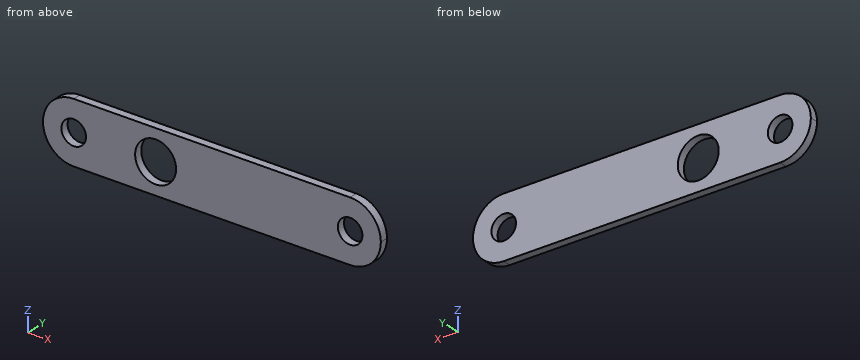
```python
from build123d import *

# Parameters (mm, degrees)
F0_W     = 82.5
F0_H     = 15
F0_R     = 3
F1_DEPTH = 1
F2_R     = 7.49999
F3_R     = 5
F4_DEPTH = 12.5


# Not quite as in the source:
# - a fillet or chamfer is up to 0.001 mm smaller than in the source, because OpenCascade refuses the exact size


with BuildPart() as f1:
    # F0 (on Front) → F1 (new body, symmetric)
    with BuildSketch(Plane.XZ):
        with Locations((33.75, 0)):
            Rectangle(F0_W, F0_H)
        Circle(F0_R, mode=Mode.SUBTRACT)
        with Locations((67.5, 0)):
            Circle(F0_R, mode=Mode.SUBTRACT)
    extrude(amount=F1_DEPTH, both=True)

    # F2 (radius 7.5 in the source; OpenCascade refuses exactly that, so slightly less here)
    f2_edges = [f1.edges().sort_by_distance(p)[0] for p in [
        (75, 0, 7.5),
        (75, 0, -7.5),
        (-7.5, 0, 7.5),
        (-7.5, 0, -7.5),
    ]]
    fillet(f2_edges, radius=F2_R)

    # F3 (on Front) → F4 (cut, symmetric)
    with BuildSketch(Plane.XZ):
        with Locations((20, 0)):
            Circle(F3_R)
    extrude(amount=F4_DEPTH, both=True, mode=Mode.SUBTRACT)


solid = f1.part
```
Check sheet for the modelled part. Datum: model origin and axes. Units: mm. Round coordinates to 2 decimals unless told otherwise and drop trailing zeros. Order: outer loops, then holes, each group sorted by start corner. A loop starts at its lowest first (then second) coordinate and runs counter-clockwise, first axis right, second up. Notation, with made-up numbers: (-6.75, 46.5) - (37.25, 46.5) arc R32 ccw to (37.25, 80.5) - close; hole circle Ø8 at (52, 3). An arc over 180 degrees is marked (long way). Answer as CSV lines item,"result". Start each with the question number.
1) Section check D-D (x = 66). Record the cut outline in (y, z), then the cut area to 3 significant figures.
2) Section check B-B (y = -0.1). Give the number of separate pieces and of enclosed holes in the cut face, then the cut area to 3 significant figures.
3) Depth check by flat-ended pin: pin 1 (1.5 mm diameter, centred on x = 16.5, z = 3.5, fed in from -Y); pin 2 (1 mm diameter, centred on y = -0.5, z = 5.5, fed in from +X). Enter the tip coordinate at first touch or a pass-through.
4) Scan lines: probe 1 along Z at (x, y) = (0, 0); probe 2 along X at (y, z) = (-0.8, 2.5); probe 3 along X at (y, z) = (0.3, 2). Record each from-to range of solid material in increasing order.
5) Section check C-C (z = -1.5). Record the cut outline in (x, y), then the cut area to 3 significant figures.
6) Section check A-A (x = 20). Record the cut outline in (y, z).
Determined:
1,outline,"(-1, -7.5) - (1, -7.5) - (1, -2.6) - (-1, -2.6) - close; (-1, 2.6) - (1, 2.6) - (1, 7.5) - (-1, 7.5) - close"
1,area,"19.6 mm^2"
2,separate pieces,"1"
2,enclosed holes,"3"
2,area,"1,050 mm^2"
3,pin 1,"y = -1"
3,pin 2,"x = 73.09"
4,probe 1,"-7.5 to -3, 3 to 7.5"
4,probe 2,"-7.07 to -1.66, 1.66 to 15.67, 24.33 to 65.84, 69.16 to 74.57"
4,probe 3,"-7.23 to -2.24, 2.24 to 15.42, 24.58 to 65.26, 69.74 to 74.73"
5,outline,"(-7.35, -1) - (-2.6, -1) - (-2.6, 1) - (-7.35, 1) - close; (2.6, -1) - (15.23, -1) - (15.23, 1) - (2.6, 1) - close; (24.77, -1) - (64.9, -1) - (64.9, 1) - (24.77, 1) - close; (70.1, -1) - (74.85, -1) - (74.85, 1) - (70.1, 1) - close"
5,area,"125 mm^2"
6,outline,"(-1, -7.5) - (1, -7.5) - (1, -5) - (-1, -5) - close; (-1, 5) - (1, 5) - (1, 7.5) - (-1, 7.5) - close"
